```python
from build123d import *

# Parameters (mm, degrees)
F1_DEPTH = 25.4
F2_DEPTH = 47.498
F3_R     = 2.54


with BuildPart() as f1:
    # F0 (on Top) → F1 (new body)
    with BuildSketch(Plane.XY):
        with BuildLine():
            ThreePointArc((8.0425684433, 27.4198416814), (22.8729864498, 17.1276710579), (28.575, 0))
            ThreePointArc((28.575, 0), (22.8729864498, -17.1276710579), (8.0425684433, -27.4198416814))
            Line((8.0425684433, -27.4198416814), (62.23, -16.3154043257))
            ThreePointArc((62.23, -16.3154043257), (75.5410049965, 0), (62.23, 16.3154043257))
            Line((62.23, 16.3154043257), (8.0425684433, 27.4198416814))
        make_face()
        with BuildLine():
            ThreePointArc((69.9632073706, 0), (62.23, -7.7332073706), (54.4967926294, 0))
            ThreePointArc((54.4967926294, 0), (62.23, 7.7332073706), (69.9632073706, 0))
        make_face(mode=Mode.SUBTRACT)
    extrude(amount=F1_DEPTH)

    # F0 (on Top) → F2 (join)
    with BuildSketch(Plane.XY):
        with BuildLine():
            ThreePointArc((8.0425684433, -27.4198416814), (22.8729864498, -17.1276710579), (28.575, 0))
            ThreePointArc((28.575, 0), (22.8729864498, 17.1276710579), (8.0425684433, 27.4198416814))
            ThreePointArc((8.0425684433, 27.4198416814), (-28.575, 0), (8.0425684433, -27.4198416814))
        make_face()
        with BuildLine():
            Line((23.5818270594, 4.3561793864), (23.5818270594, 0))
            Line((23.5818270594, 0), (23.5818270594, -4.3561793864))
            Line((23.5818270594, -4.3561793864), (15.2656256391, -4.3561793864))
            ThreePointArc((15.2656256391, -4.3561793864), (-15.875, 0), (15.2656256391, 4.3561793864))
            Line((15.2656256391, 4.3561793864), (23.5818270594, 4.3561793864))
        make_face(mode=Mode.SUBTRACT)
    extrude(amount=F2_DEPTH)

    # F3
    f3_edges = [f1.edges().sort_by_distance(p)[0] for p in [
        (-8.042568, 27.419842, 47.498),
    ]]
    fillet(f3_edges, radius=F3_R)


solid = f1.part
```
Build history of the part. All positions in model axes, mm. A direction names the side the tool comes from. Give positions to 0.01 mm unless a question says otherwise; leave off trailing zeros. Order: outer loops, then holes, each group sorted by start corner. A loop starts at its lowest first (then second) coordinate and runs counter-clockwise, first axis right, second up. Notation, with made-up numbers: M 7.5,-15 L 42.5,-15 A18 cw 42.5,6 Z; hole C 30,11 d5. An arc over 180 degrees is marked long. Write item = value, one per line. Start each with the question number.
(1) Slice it at B-B on x = 65.5. Write the cut outline in (y, z).
(2) Slice it at D-D on y = 6. State how many separate pieces and enclosed holes the cut face has, plus the area to 3 significant figures.
(3) Which spindle directions (+Z, -Z, +X, -X, +Y, -Y) get a long thin tool onto all of the face, cutting with end or side? Do faces 1 (the flat face through (-12, -11, 47.498)), 2 (the flat face through (23.582, 0, 23)). Say none if no direction does.
(4) Slice it at C-C on z = 11.5. Write the cut outline in (x, y) (3 decimals), plus the area to 3 significant figures.
(5) Slice it at A-A on z = 33. Write the cut outline in (x, y) (3 decimals).
(6) Probe L1, parallel to Y at x = 62.23, z = 17; L2, parallel to Y at x = 0.5, z = 10.5; L3, parallel to X at y = -1, z = 2. List the from-to ranges inside material, lowest first. Write a range as [from, to].
(7) Pin check, flat tips, straight feed: pin 1 Ø2.5 at (x, z) = (19, 16.5) entering from -Y; pin 2 Ø6.5 at (x, z) = (20.5, 35.5) entering from +Y; pin 3 Ø4 at (y, z) = (13, 25.5) entering from +X. Stop position of each tip, or through.
Responses:
q1.outline = M -15.29,0 L -7.01,0 L -7.01,25.4 L -15.29,25.4 Z; M 7.01,0 L 15.29,0 L 15.29,25.4 L 7.01,25.4 Z
q2.separate_pieces = 3
q2.enclosed_holes = 0
q2.area = 2,190 mm2
q3.face_1 = +Z, +X, -X, +Y, -Y
q3.face_2 = +Z, -Z
q4.outline = M 8.043,-27.42 L 62.23,-16.315 A16.654 ccw 62.23,16.315 L 8.043,27.42 A28.575 ccw long Z; hole M 15.266,-4.356 L 23.582,-4.356 L 23.582,4.356 L 15.266,4.356 A15.875 ccw long Z; hole C 62.23,0 d15.466
q4.area = 3,380 mm2
q5.outline = C 0,0 d57.15; hole M 15.266,-4.356 L 23.582,-4.356 L 23.582,4.356 L 15.266,4.356 A15.875 ccw long Z
q6.L1 = [-16.32, -7.73], [7.73, 16.32]
q6.L2 = [-28.57, -15.87], [15.87, 28.57]
q6.L3 = [-28.56, -15.84], [23.58, 54.56], [69.9, 75.51]
q7.pin_1 = -25.43
q7.pin_2 = 22.78
q7.pin_3 = 71.39
